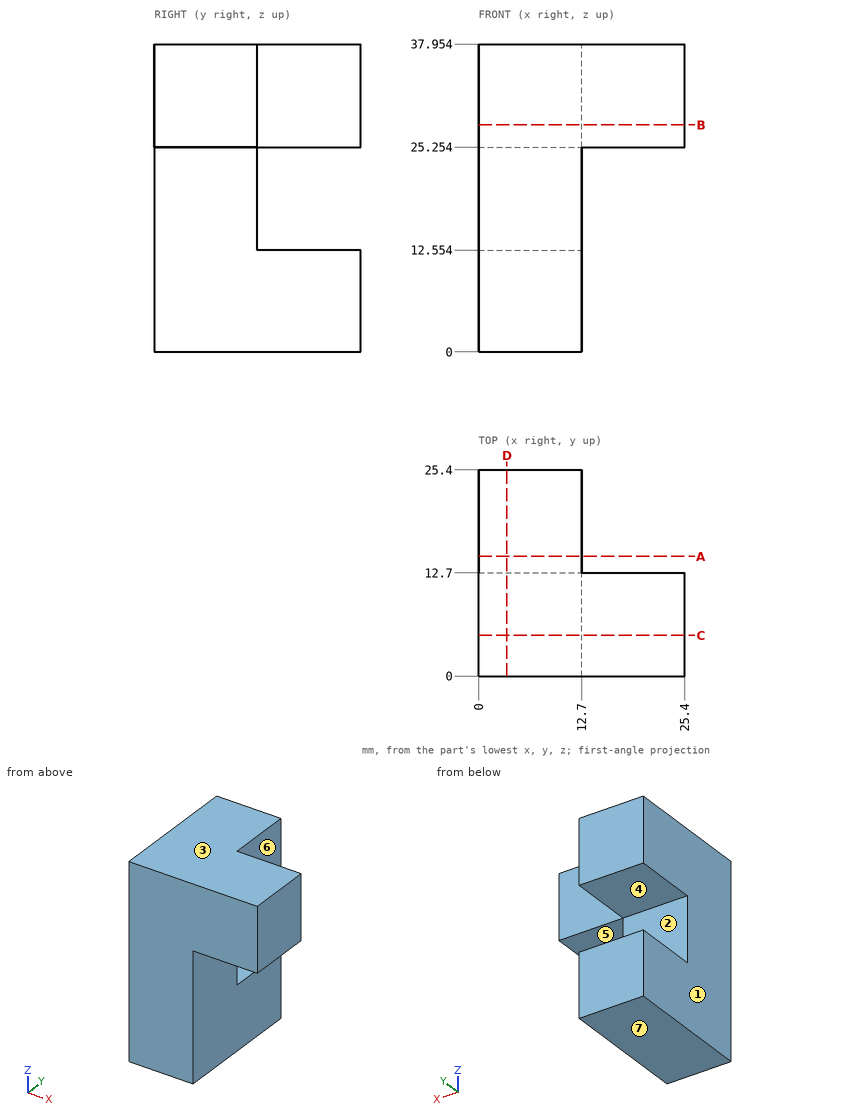
Design review of the part shown in the three views and the two pictorial views. Dimensions are in mm from the part's minimum x, y and z. A direction names the side the tool comes from. Coordinates: 2 decimals unless noted, no trailing zeros. Loops run counter-clockwise (first coordinate to the right, second up) from the corner with the lowest first, then second, coordinate; pieces in that order, holes last.
Q1. We need section B-B on z = 28. State the section outline as (x, y) points, and give its area (3 significant figures).
Reported:
outline: (0, 0) - (25.4, 0) - (25.4, 12.7) - (12.7, 12.7) - (12.7, 25.4) - (0, 25.4) - close
area: 484 mm2
Q2. We need section D-D on x = 3.5. State the section outline as (y, z) points, and give its area (3 significant figures).
Reported:
outline: (0, 0) - (25.4, 0) - (25.4, 12.55) - (12.7, 12.55) - (12.7, 25.25) - (25.4, 25.25) - (25.4, 37.95) - (0, 37.95) - close
area: 803 mm2
Q3. We need section A-A on y = 14.75. State the section outline as (x, z) points.
Reported:
outline: (0, 0) - (12.7, 0) - (12.7, 12.55) - (0, 12.55) - close; (0, 25.25) - (12.7, 25.25) - (12.7, 37.95) - (0, 37.95) - close
Q4. For pin 1 (6.5 mm diameter, centred on x = 8, z = 17, fed in from +Y); pin 2 (6 mm diameter, centred on y = 4.5, z = 20, fed in from +X); pin 3 (4 mm diameter, centred on x = 20, y = 8.5, fed in from -Z), all flat-tipped, find the tip position at first contact; note any pin that passes through.
Reported:
pin 1: stops at y = 12.7
pin 2: stops at x = 12.7
pin 3: stops at z = 25.25
Q5. Tool access review of the marked faces 5, 6 and 7: name each direction out of +Z, -Z, +X, -X, +Y, -Y from which nothing blocks a thin tool from reaching the whole face with its end or side.
Reported:
face 5: -Z, +X, +Y, -Y
face 6: +Z, -Z, +X, +Y
face 7: -Z, +X, -X, +Y, -Y
Q6. The part is to be moulded in two halves that separate along Z. For the marked faces 1, 2, 3 and 4, say which applies: +Z half, -Z half, draft (parallel to the pull), parting line (faces both ways), or undercut.
Reported:
face 1: draft
face 2: undercut
face 3: +Z half
face 4: undercut
Q7. To check wall thickness, follow line 1 (Z direction, x = 3.5, y = 14); line 2 (X direction, y = 12.25, z = 21); line 3 (Z direction, x = 19, y = 9). State the ranges of each line that lie inside material, in increasing order.
Reported:
line 1: z = 0 to 12.55, 25.25 to 37.95
line 2: x = 0 to 12.7
line 3: z = 25.25 to 37.95
Q8. We need section C-C on y = 5. State the section outline as (x, z) points, and give its area (3 significant figures).
Reported:
outline: (0, 0) - (12.7, 0) - (12.7, 25.25) - (25.4, 25.25) - (25.4, 37.95) - (0, 37.95) - close
area: 643 mm2
